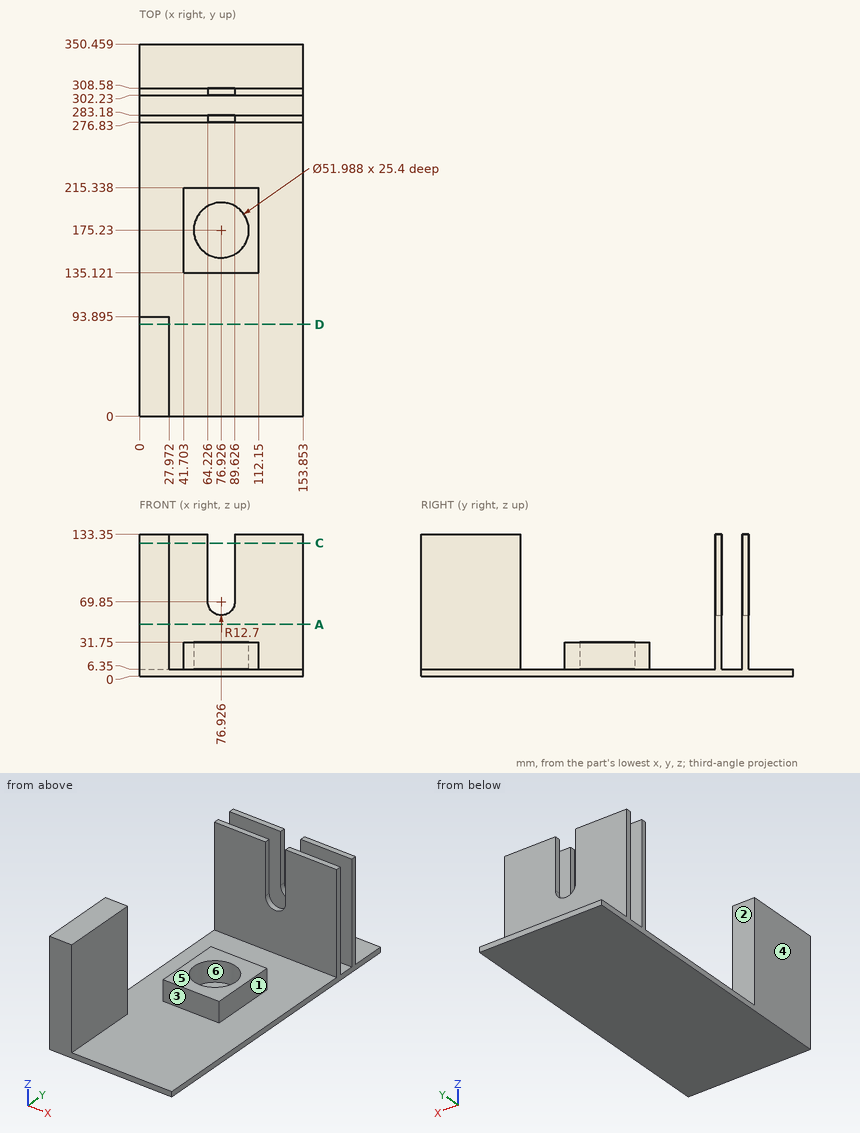
Study the drawing (mm; zero at the part's minimum x, y, z) and answer. A direction names the side the tool comes from. Coordinates: 2 decimals unless noted, no trailing zeros. Write each loop counter-clockwise with the first axis right and the second up, starting at its lowest first coordinate (ties: lowest second). Pieces come first, ordered by that corner, then holes. Notation, with made-up numbers: (86.5, 34) - (132.5, 34) arc R26 ccw to (132.5, 66) - close; hole circle Ø9 at (-33.75, -18). An arc over 180 degrees is marked (long way). Return JSON: item names as keys, results as strings. Group by question number.
1. A cutting plane is placed at D-D, the plane y = 86.5. Determine the outline of the cut face in (x, z), plus the area to 3 significant figures.
2. Given pin 1 (12 mm diameter, centred on x = 128.5, y = 223.5, fed in from +Z); pin 2 (8.5 mm diameter, centred on x = 16.5, z = 71.5, fed in from +Y); pin 3 (12 mm diameter, centred on x = 123, z = 98, fed in from -Y), each flat-ended and moving along its own axis, determine where each tip first touches the part or whether it passes through.
3. A cutting plane is placed at C-C, the plane z = 125. Determine the outline of the cut face in (x, y) (1 decimal), plus the area to 3 significant figures.
4. A cutting plane is placed at A-A, the plane z = 48.5. Determine the outline of the cut face in (x, y) (1 decimal), plus the area to 3 significant figures.
5. Which of the six approach directions +Z, -Z, +X, -X, +Y, -Y give full straight-line access (tool end or side, diameter ignored) to the marked faces 1, 2 and 3?
6. Determine the mould class of the marked faces 4, 5 and 6 for opening direction X: released by +X, released by -X, zero draft, split by the parting line, or undercut.
7. Straight lines are drawn through the part: L1, parallel to Y at x = 7, z = 124.5 (1 decimal); L2, parallel to X at y = 54.5, z = 53.5; L3, parallel to Z at x = 36, y = 141. For each, find the intervals that lie inside material, in ascending order.
Ans:
{
 "1": {"outline": "(0, 0) - (153.85, 0) - (153.85, 6.35) - (27.97, 6.35) - (27.97, 133.35) - (0, 133.35) - close", "area": "4,530 mm²"},
 "2": {"pin 1": "z = 6.35", "pin 2": "y = 308.58", "pin 3": "y = 276.83"},
 "3": {"outline": "(0, 0) - (28, 0) - (28, 93.9) - (0, 93.9) - close; (0, 276.8) - (64.2, 276.8) - (64.2, 283.2) - (0, 283.2) - close; (0, 302.2) - (64.2, 302.2) - (64.2, 308.6) - (0, 308.6) - close; (89.6, 276.8) - (153.9, 276.8) - (153.9, 283.2) - (89.6, 283.2) - close; (89.6, 302.2) - (153.9, 302.2) - (153.9, 308.6) - (89.6, 308.6) - close", "area": "4,260 mm²"},
 "4": {"outline": "(0, 0) - (28, 0) - (28, 93.9) - (0, 93.9) - close; (0, 276.8) - (153.9, 276.8) - (153.9, 283.2) - (0, 283.2) - close; (0, 302.2) - (153.9, 302.2) - (153.9, 308.6) - (0, 308.6) - close", "area": "4,580 mm²"},
 "5": {"face 1": "+Z, +X, -Y", "face 2": "+Z, +X, -X", "face 3": "+Z, +X, -X, -Y"},
 "6": {"face 4": "released by -X", "face 5": "zero draft", "face 6": "undercut"},
 "7": {"L1": "0 to 93.9, 276.8 to 283.2, 302.2 to 308.6", "L2": "0 to 27.97", "L3": "0 to 6.35"}
}
